Here's how the part is built. I have some questions about the finished solid (model axes, mm). Give positions to 0.01 mm unless a question says otherwise; leave off trailing zeros. Write each loop counter-clockwise with the first axis right and the second up, starting at its lowest first coordinate (ties: lowest second). Pieces come first, ordered by that corner, then holes. Notation, with made-up numbers: (38, -12) - (71, -12) arc R6 cw to (71, -2) - close; hole circle Ø8 at (82, 53). An arc over 180 degrees is marked (long way). Use a Markdown table: item, result.
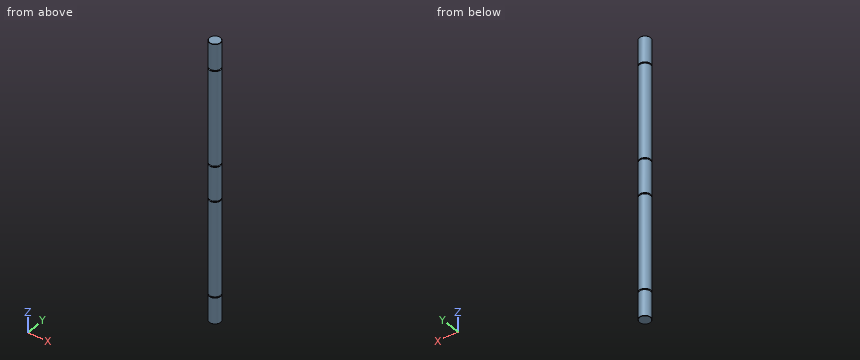
```python
from build123d import *

# Parameters (mm, degrees)
SKETCH2_R                = 3
BOSS_EXTRUDE1_DEPTH      = 75
BOSS_EXTRUDE1_DEPTH_BACK = 75
CHAMFER1_SIZE            = 0.12
CUT_EXTRUDE1_START       = -13.936057366
SKETCH3_R                = 3
SKETCH3_R_2              = 2.5
CUT_EXTRUDE1_DEPTH       = 0.7
CUT_EXTRUDE2_START       = -65.26
SKETCH3_2_R              = 3
SKETCH3_2_R_2            = 2.5
CUT_EXTRUDE2_DEPTH       = 0.7


with BuildPart() as part:
    # Sketch2 → Boss-Extrude1 (new body, two sides)
    with BuildSketch(Plane.XY) as boss_extrude1_sk:
        Circle(SKETCH2_R)
    extrude(amount=BOSS_EXTRUDE1_DEPTH)
    extrude(boss_extrude1_sk.sketch, amount=-BOSS_EXTRUDE1_DEPTH_BACK)

    # Chamfer1
    chamfer1_edges = [part.edges().sort_by_distance(p)[0] for p in [
        (-3, 0, -75),
        (-3, 0, 75),
    ]]
    chamfer(chamfer1_edges, length=CHAMFER1_SIZE)

    # Sketch3 → Cut-Extrude1 (cut)
    with BuildSketch(Plane.XY.offset(75).offset(CUT_EXTRUDE1_START)):
        Circle(SKETCH3_R)
        Circle(SKETCH3_R_2, mode=Mode.SUBTRACT)
    cut_extrude1 = extrude(amount=-CUT_EXTRUDE1_DEPTH, mode=Mode.SUBTRACT)

    # Mirror1: Cut-Extrude1 across plane
    add(cut_extrude1.mirror(Plane.XY), mode=Mode.SUBTRACT)

    # Sketch3<2> → Cut-Extrude2 (cut)
    with BuildSketch(Plane.XY.offset(75).offset(CUT_EXTRUDE2_START)):
        Circle(SKETCH3_2_R)
        Circle(SKETCH3_2_R_2, mode=Mode.SUBTRACT)
    cut_extrude2 = extrude(amount=-CUT_EXTRUDE2_DEPTH, mode=Mode.SUBTRACT)

    # Mirror2: Cut-Extrude2 across plane
    add(cut_extrude2.mirror(Plane.XY), mode=Mode.SUBTRACT)


solid = part.part
```
Item 1: Will these pins go through, and if not, where does the flat tip stop? pin 1 Ø2 at (x, z) = (1, 50.5) entering from -Y; pin 2 Ø1 at (y, z) = (1.5, -55.5) entering from -X.
Values:
| item | result |
|---|---|
| pin 1 | stops at y = -3 |
| pin 2 | stops at x = -2.83 |
Item 2: If we section it at A-A, the plane z = -42.5: Write out the boundary of the cut face in (x, y), plus the area to 3 significant figures.
Values:
| item | result |
|---|---|
| outline | circle Ø6 at (0, 0) |
| area | 28.3 mm2 |
Item 3: I need wall thicknesses on line 1 along Z through (x, y) = (-0.95, -2.35); line 2 along X through (y, z) = (0.3, 41); line 3 along Y through (x, z) = (-0.15, 13). Which ranges of each line are inside material? Lowest first, please. Write a range as [from, to].
Values:
| item | result |
|---|---|
| line 1 | z = [-75, -61.06], [-60.36, -9.74], [-9.04, 9.04], [9.74, 60.36], [61.06, 75] |
| line 2 | x = [-2.98, 2.98] |
| line 3 | y = [-3, 3] |
